```python
from build123d import *

# Parameters (mm, degrees)
F0_R     = 40
F0_R_2   = 2.5
F1_DEPTH = 10


with BuildPart() as f1:
    # F0 (on Front) → F1 (new body)
    with BuildSketch(Plane.XZ):
        Circle(F0_R)
        with BuildLine():
            Line((-30.5941170816, -5), (-5.5901699437, -5))
            ThreePointArc((-5.5901699437, -5), (-5.3033008589, -5.3033008589), (-5, -5.5901699437))
            Line((-5, -5.5901699437), (-5, -30.5941170816))
            ThreePointArc((-5, -30.5941170816), (-21.9203102168, -21.9203102168), (-30.5941170816, -5))
        make_face(mode=Mode.SUBTRACT)
        with BuildLine():
            ThreePointArc((5, -5.5901699437), (5.3033008589, -5.3033008589), (5.5901699437, -5))
            Line((5.5901699437, -5), (30.5941170816, -5))
            ThreePointArc((30.5941170816, -5), (21.9203102168, -21.9203102168), (5, -30.5941170816))
            Line((5, -30.5941170816), (5, -5.5901699437))
        make_face(mode=Mode.SUBTRACT)
        with BuildLine():
            ThreePointArc((-30.5941170816, 5), (-21.9203102168, 21.9203102168), (-5, 30.5941170816))
            Line((-5, 30.5941170816), (-5, 5.5901699437))
            ThreePointArc((-5, 5.5901699437), (-5.3033008589, 5.3033008589), (-5.5901699437, 5))
            Line((-5.5901699437, 5), (-30.5941170816, 5))
        make_face(mode=Mode.SUBTRACT)
        Circle(F0_R_2, mode=Mode.SUBTRACT)
        with BuildLine():
            Line((30.5941170816, 5), (5.5901699437, 5))
            ThreePointArc((5.5901699437, 5), (5.3033008589, 5.3033008589), (5, 5.5901699437))
            Line((5, 5.5901699437), (5, 30.5941170816))
            ThreePointArc((5, 30.5941170816), (21.9203102168, 21.9203102168), (30.5941170816, 5))
        make_face(mode=Mode.SUBTRACT)
    extrude(amount=F1_DEPTH)


solid = f1.part
```
Read the model definition and answer for the solid it produces. Units are mm, in the model's axes. A direction names the side the tool comes from. Coordinates: 2 decimals unless noted, no trailing zeros. Write each loop counter-clockwise with the first axis right and the second up, starting at its lowest first coordinate (ties: lowest second). Pieces come first, ordered by that corner, then holes. Notation, with made-up numbers: (-20.75, 47.5) -> (13.25, 47.5) arc R32 ccw to (13.25, 77.5) -> close; hole circle Ø2 at (48, 78.25). An arc over 180 degrees is marked (long way). Write item = value, one per line.
(1) For a pull along Z with two mould halves and no side action, classify faces 1 (the face through (22.11, -4.93, -21.73)), 2 (the face through (-8.67, -4.93, -39.05)), 3 (the face through (-1, -10, -8)) as +Z half, -Z half, draft (parallel to the pull), parting line (faces both ways), or undercut.
From the geometry:
face_1 = undercut
face_2 = parting line
face_3 = draft
(2) Section D-D on x = -14 is taken. Write down the section's boundary in (y, z).
From the geometry:
outline = (-10, -37.47) -> (0, -37.47) -> (0, -27.66) -> (-10, -27.66) -> close; (-10, -5) -> (0, -5) -> (0, 5) -> (-10, 5) -> close; (-10, 27.66) -> (0, 27.66) -> (0, 37.47) -> (-10, 37.47) -> close
(3) Given pin 1 Ø2 at (y, z) = (-6.5, 29) entering from -X; pin 2 Ø5 at (x, y) = (-18.5, -6) entering from +Z; pin 3 Ø1.5 at (y, z) = (-6, -13) entering from +X, each flat-ended and moving along its own axis, determine where each tip first touches the part or whether it passes through.
From the geometry:
pin_1 = -28.57
pin_2 = 36.66
pin_3 = 38.08
(4) Which of the six approach directions +Z, -Z, +X, -X, +Y, -Y give full straight-line access (tool end or side, diameter ignored) to faces 4 (the face through (18, -5, 5)), 5 (the face through (-1, 0, -8))?
From the geometry:
face_4 = +Y, -Y
face_5 = +Z, -Z, +X, -X, +Y
(5) Straight lines are drawn through the part: L1, parallel to Z at x = 0, y = -1.75; L2, parallel to Z at x = 13.5, y = -9.5; L3, parallel to X at y = -4.25, z = -12. For each, find the intervals that lie inside material, in ascending order. Write a range as from..to.
From the geometry:
L1 = -40..-2.5, 2.5..40
L2 = -37.65..-27.91, -5..5, 27.91..37.65
L3 = -38.16..-28.58, -5..5, 28.58..38.16
(6) Section B-B on z = 7 is taken. Write down the section's boundary in (x, y).
From the geometry:
outline = (-39.38, -10) -> (-30.2, -10) -> (-30.2, 0) -> (-39.38, 0) -> close; (-5, -10) -> (5, -10) -> (5, 0) -> (-5, 0) -> close; (30.2, -10) -> (39.38, -10) -> (39.38, 0) -> (30.2, 0) -> close
(7) Section A-A on x = 0 is taken. Write down the section's boundary in (y, z).
From the geometry:
outline = (-10, -40) -> (0, -40) -> (0, -2.5) -> (-10, -2.5) -> close; (-10, 2.5) -> (0, 2.5) -> (0, 40) -> (-10, 40) -> close
(8) Section C-C on y = -2.5 is taken. Write down the section's boundary in (x, z), plus the area to 3 significant figures.
From the geometry:
outline = circle Ø80 at (0, 0); hole (-30.59, -5) arc R31 ccw to (-5, -30.59) -> (-5, -5.59) arc R7.5 cw to (-5.59, -5) -> close; hole (-30.59, 5) -> (-5.59, 5) arc R7.5 cw to (-5, 5.59) -> (-5, 30.59) arc R31 ccw to start; hole circle Ø5 at (0, 0); hole (5, -30.59) arc R31 ccw to (30.59, -5) -> (5.59, -5) arc R7.5 cw to (5, -5.59) -> close; hole (5, 5.59) arc R7.5 cw to (5.59, 5) -> (30.59, 5) arc R31 ccw to (5, 30.59) -> close
area = 3,120 mm2
